Geometry check sheet. Reference: the model listing, model coordinates, mm. A direction names the side the tool comes from. Coordinates: 2 decimals unless noted, no trailing zeros. Order: outer loops, then holes, each group sorted by start corner. A loop starts at its lowest first (then second) coordinate and runs counter-clockwise, first axis right, second up. Notation, with made-up numbers: (15, 61) - (19, 61) arc R21 ccw to (19, 89) - close; hole circle Ø5 at (31.5, -34.5). An arc over 180 degrees is marked (long way). Return JSON: item names as keys, results as strings. Group by question number.
Item 1: Draft check along Z on faces 4 (the flat face through (0, 30, 0)), 5 (the flat face through (-8, 0, -8)), 6 (the cylindrical face through (-10.344, 114.624, 1.825)). Enter one of: pulls with the +Z half, pulls with the -Z half, needs draft (parallel to the pull), parting line crosses it, or undercut.
Item 2: Gauge pin test, flat ends, axial feed: pin 1 (4 mm diameter, centred on x = -8, z = 6, fed in from +Y); pin 2 (1.5 mm diameter, centred on x = 4, y = 41.5, fed in from -Z); pin 3 (4 mm diameter, centred on x = -11.5, z = 8.5, fed in from -Y); pin 4 (1 mm diameter, centred on x = 13.5, z = 15, fed in from -Y). Record the tip position at first contact, or that the pin passes through.
Item 3: Tool access check on faces 1 (the cylindrical face through (-2.17, 14.79, -9.76)), 2 (the cylindrical face through (-4.336, 6.01, -19.524)), 3 (the flat face through (4, 56, -4)). Record the directions out of +Z, -Z, +X, -X, +Y, -Y that give a thin tool (end or side, any length) a straight path to the whole face; none if there is none.
Item 4: Section check A-A on y = 24. Enter the section's corners in (x, z).
Item 5: Scan lines: probe 1 along Z at (x, y) = (0, 8.75); probe 2 along Z at (x, y) = (0, 18); probe 3 along Y at (x, z) = (-0.5, 6). Record each from-to range of solid material in increasing order.
from build123d import *

# Parameters (mm, degrees)
SKETCH4_R = 3
FILLET1_R = 2


with BuildPart() as part:
    # Sketch1 → Revolve1 (revolve)
    with BuildSketch(Plane.XY):
        Polygon((10, 0), (20, 0), (20, 10.125), (10, 56), (0, 56), (0, 30), (10, 30), align=None)
    revolve(axis=Axis((0, 42, 0), (0, -1, 0)))

    # Sweep1: sweep along a path in Sketch2
    with BuildLine(Plane.XY) as sweep1_path:
        Line((0, 56), (0, 95.080892972))
        ThreePointArc((0, 95.080892972), (-1.809221376, 105.341497272), (-7.018666706, 114.364521263))
        Line((-7.018666706, 114.364521263), (-10.284601755, 118.25671109))
    # Sketch4 → Sweep1 (sweep)
    with BuildSketch(Plane(origin=(0, 56, 0), x_dir=(1, 0, 0), z_dir=(0, 1, 0))):
        Circle(SKETCH4_R)
    sweep(path=sweep1_path.line)

    # Sketch3 → Revolve2 (revolve)
    with BuildSketch(Plane.XY):
        Polygon((-10.284601755, 118.25671109), (-7.986468426, 120.185073919), (-14.141327413, 122.852977749), align=None)
    revolve(axis=Axis((-14.141327413, 122.852977749, 0), (0.64278761, -0.766044443, 0)))

    # Fillet1
    fillet1_edges = [part.edges().sort_by_distance(p)[0] for p in [
        (-3, 56, 0),
        (-12.582735084, 116.328348261, 0),
        (-10, 56, 0),
        (-20, 10.125, 0),
        (-20, 0, 0),
    ]]
    fillet(fillet1_edges, radius=FILLET1_R)


solid = part.part
Computed:
{
 "1": {"face 4": "undercut", "face 5": "needs draft", "face 6": "parting line crosses it"},
 "2": {"pin 1": "stops at y = 56", "pin 2": "stops at z = -12.82", "pin 3": "stops at y = 0", "pin 4": "stops at y = 0.92"},
 "3": {"face 1": "-Y", "face 2": "+Y, -Y", "face 3": "none"},
 "4": {"outline": "circle Ø33.95 at (0, 0); hole circle Ø20 at (0, 0)"},
 "5": {"probe 1": "z = -20 to -10, 10 to 20", "probe 2": "z = -18.28 to -10, 10 to 18.28", "probe 3": "y = 30 to 56"}
}
